Can you work these out from the drawing? Everything is in mm from the part's minimum corner. Coordinates: 2 decimals unless noted, no trailing zeros. Loops run counter-clockwise (first coordinate to the right, second up) from the corner with the lowest first, then second, coordinate; pieces in that order, holes last.
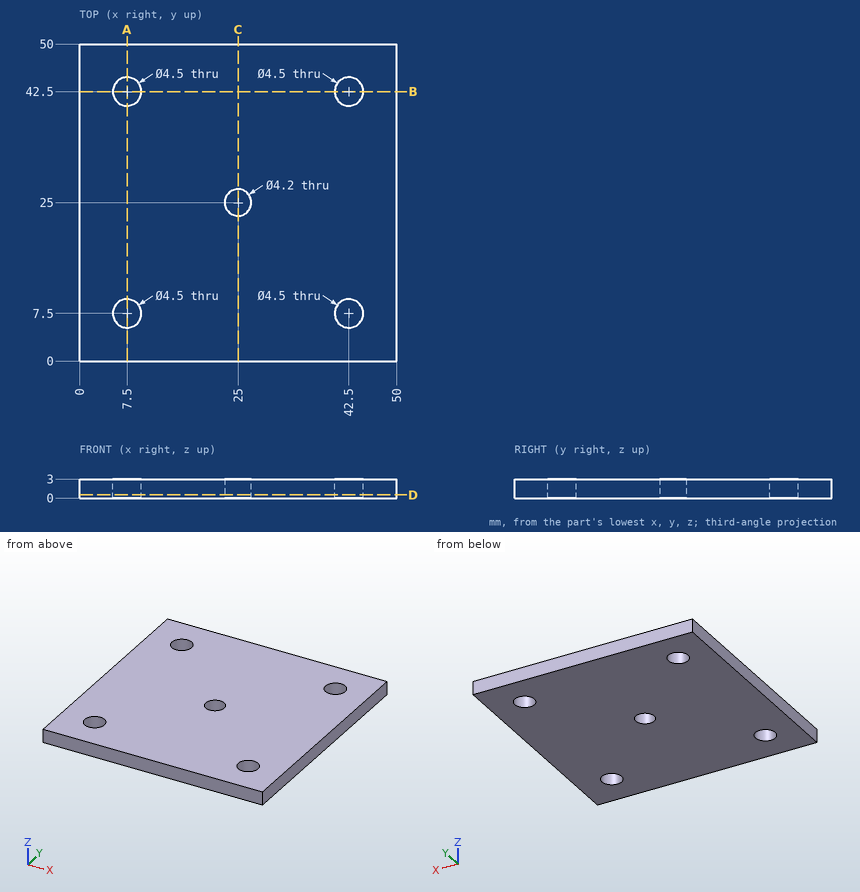
1) Imagine slicing it at D-D on z = 0.5. List the corners of the cut face in (x, y) for me.
2) If I drill on L1, parallel to Y at x = 42.5, z = 0.7; L2, parallel to Y at x = 25, z = 1.8, over which ranges is the centre line in solid material (lowest first)?
3) Imagine slicing it at C-C on x = 25. List the corners of the cut face in (y, z) for me, plus the area to 3 significant figures.
4) Will these pins go through, and if not, where does the flat tip stop? pin 1 (3.5 mm diameter, centred on x = 25, y = 25, fed in from +Z); pin 2 (5 mm diameter, centred on x = 42.5, y = 7.5, fed in from +Z).
5) Imagine slicing it at A-A on x = 7.5. List the corners of the cut face in (y, z) for me, plus the area to 3 significant figures.
Solved:
1. outline: (0, 0) - (50, 0) - (50, 50) - (0, 50) - close; hole circle Ø4.5 at (7.5, 7.5); hole circle Ø4.5 at (7.5, 42.5); hole circle Ø4.2 at (25, 25); hole circle Ø4.5 at (42.5, 7.5); hole circle Ø4.5 at (42.5, 42.5)
2. L1: y = 0 to 5.25, 9.75 to 40.25, 44.75 to 50
2. L2: y = 0 to 22.9, 27.1 to 50
3. outline: (0, 0) - (22.9, 0) - (22.9, 3) - (0, 3) - close; (27.1, 0) - (50, 0) - (50, 3) - (27.1, 3) - close
3. area: 137 mm2
4. pin 1: passes through
4. pin 2: stops at z = 3
5. outline: (0, 0) - (5.25, 0) - (5.25, 3) - (0, 3) - close; (9.75, 0) - (40.25, 0) - (40.25, 3) - (9.75, 3) - close; (44.75, 0) - (50, 0) - (50, 3) - (44.75, 3) - close
5. area: 123 mm2
